from build123d import *

# Parameters (mm, degrees)
F2_R     = 1.75
F3_DEPTH = 25


with BuildPart() as f1:
    # F0 (on Front) → F1 (revolve)
    with BuildSketch(Plane.XZ):
        Polygon((5.125, 1.85), (3.5, 1.85), (3.5, -13.75), (5.125, -13.75), (5.125, -3.6), (11.125, -3.6), (11.125, 0), (5.125, 0), align=None)
    revolve(axis=Axis((0, 0, -12.131187), (0, 0, -1)))

    # F2 (on face) → F3 (cut)
    with BuildSketch(Plane.XY):
        with Locations((0, 8)):
            Circle(F2_R)
        with Locations((-8, 0)):
            Circle(F2_R)
        with Locations((0, -8)):
            Circle(F2_R)
        with Locations((8, 0)):
            Circle(F2_R)
    extrude(amount=-F3_DEPTH, mode=Mode.SUBTRACT)


solid = f1.part
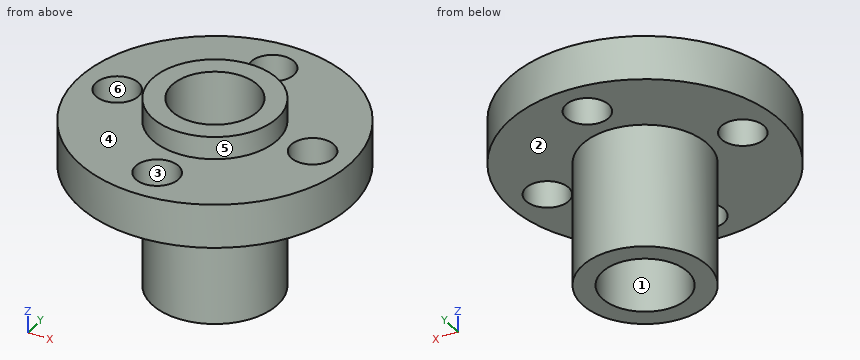
Could you check a few things on this model? Use its own coordinates, in mm. Face numbers are marked on the shaded views. A direction names the side the tool comes from. Coordinates: 2 decimals unless noted, no trailing zeros. Loops run counter-clockwise (first coordinate to the right, second up) from the corner with the lowest first, then second, coordinate; pieces in that order, holes last. Notation, with made-up numbers: (-18.75, 7) -> (-8.75, 7) arc R17 ccw to (-8.75, 39) -> close; hole circle Ø3 at (51, 28.25). An arc over 180 degrees is marked (long way). Answer in a Markdown table with one row per item.
(1) Will these pins go through, and if not, where does the flat tip stop? pin 1 Ø2 at (x, z) = (-1.5, -6) entering from -Y; pin 2 Ø3 at (y, z) = (5, 0) entering from +X; pin 3 Ø4 at (x, y) = (0, 8) entering from +Z.
Results found:
| item | result |
|---|---|
| pin 1 | stops at y = -5.1 |
| pin 2 | stops at x = 10.56 |
| pin 3 | stops at z = 0 |
(2) Imagine slicing it at A-A (y = 0). List the corners of the cut face in (x, z) for me (3 decimals), plus the area to 3 significant figures.
Results found:
| item | result |
|---|---|
| outline | (-11.125, -3.6) -> (-9.75, -3.6) -> (-9.75, 0) -> (-11.125, 0) -> close; (-6.25, -3.6) -> (-5.125, -3.6) -> (-5.125, -13.75) -> (-3.5, -13.75) -> (-3.5, 1.85) -> (-5.125, 1.85) -> (-5.125, 0) -> (-6.25, 0) -> close; (3.5, -13.75) -> (5.125, -13.75) -> (5.125, -3.6) -> (6.25, -3.6) -> (6.25, 0) -> (5.125, 0) -> (5.125, 1.85) -> (3.5, 1.85) -> close; (9.75, -3.6) -> (11.125, -3.6) -> (11.125, 0) -> (9.75, 0) -> close |
| area | 68.7 mm^2 |
(3) For the marked faces 1 and 2, which set-ups out of +Z, -Z, +X, -X, +Y, -Y let a thin tool reach every point of the face, with its end or its side?
Results found:
| item | result |
|---|---|
| face 1 | +Z, -Z |
| face 2 | -Z |
(4) Thinking about a two-plate mould opening in Y: for the marked faces 3, 4, 5 and 6, which applies, released by +Y, released by -Y, zero draft, split by the parting line, or undercut?
Results found:
| item | result |
|---|---|
| face 3 | undercut |
| face 4 | zero draft |
| face 5 | split by the parting line |
| face 6 | undercut |
(5) Imagine slicing it at B-B (x = -7.5). List the corners of the cut face in (y, z) for me.
Results found:
| item | result |
|---|---|
| outline | (-8.22, -3.6) -> (-1.68, -3.6) -> (-1.68, 0) -> (-8.22, 0) -> close; (1.68, -3.6) -> (8.22, -3.6) -> (8.22, 0) -> (1.68, 0) -> close |
(6) Imagine slicing it at D-D (y = 8.75). List the corners of the cut face in (x, z) for me, plus the area to 3 significant figures.
Results found:
| item | result |
|---|---|
| outline | (-6.87, -3.6) -> (-1.58, -3.6) -> (-1.58, 0) -> (-6.87, 0) -> close; (1.58, -3.6) -> (6.87, -3.6) -> (6.87, 0) -> (1.58, 0) -> close |
| area | 38.1 mm^2 |
(7) If I drill on probe 1 along Y at (x, z) = (0, -1.3) (3 decimals); probe 2 along Y at (x, z) = (8, -2.75); probe 3 along X at (y, z) = (1.75, -4.75), over which ranges is the centre line in solid material (lowest first)?
Results found:
| item | result |
|---|---|
| probe 1 | y = -11.125 to -9.75, -6.25 to -3.5, 3.5 to 6.25, 9.75 to 11.125 |
| probe 2 | y = -7.73 to -1.75, 1.75 to 7.73 |
| probe 3 | x = -4.82 to -3.03, 3.03 to 4.82 |
